```python
from build123d import *

# Parameters (mm, degrees)
F0_R     = 5.375
F0_R_2   = 2.6
F1_DEPTH = 3
F2_DEPTH = 1


with BuildPart() as f1:
    # F0 (on Top) → F1 (new body)
    with BuildSketch(Plane.XY):
        with BuildLine():
            Line((75, 10), (0, 10))
            ThreePointArc((0, 10), (-10, 0), (0, -10))
            Line((0, -10), (75, -10))
            ThreePointArc((75, -10), (85, 0), (75, 10))
        make_face()
        Circle(F0_R, mode=Mode.SUBTRACT)
        with Locations((75, 0)):
            Circle(F0_R, mode=Mode.SUBTRACT)
        with Locations((75, 0)):
            Circle(F0_R)
        with Locations((75, 0)):
            Circle(F0_R_2, mode=Mode.SUBTRACT)
        Circle(F0_R)
        Circle(F0_R_2, mode=Mode.SUBTRACT)
    extrude(amount=-F1_DEPTH)

    # F0 (on Top) → F2 (cut)
    with BuildSketch(Plane.XY):
        with Locations((75, 0)):
            Circle(F0_R)
        with Locations((75, 0)):
            Circle(F0_R_2, mode=Mode.SUBTRACT)
        Circle(F0_R)
        Circle(F0_R_2, mode=Mode.SUBTRACT)
    extrude(amount=-F2_DEPTH, mode=Mode.SUBTRACT)


solid = f1.part
```
Work out the finished part from the listing and answer in its coordinate system (mm). A direction names the side the tool comes from. Coordinates: 2 decimals unless noted, no trailing zeros. Write each loop counter-clockwise with the first axis right and the second up, starting at its lowest first coordinate (ties: lowest second). Pieces come first, ordered by that corner, then holes.
Q1. A cutting plane is placed at C-C, the plane x = 76. Give the vertices of the cut face in (y, z).
Q2. Determine the mould class of faces 1 (the face through (-10, 0, -1)), 2 (the face through (37, -10, -1)), 3 (the face through (-0.7, 5.33, -0.49)), 4 (the face through (80.13, 1.61, -0.49)) for opening direction X: released by +X, released by -X, zero draft, split by the parting line, or undercut.
Q3. Find the intervals of material crossed by line 1 (X direction, y = 1, z = -1.7); line 2 (Y direction, x = 0, z = -2.2); line 3 (Y direction, x = 0, z = -0.3) (3 decimals), in increasing order.
Q4. A cutting plane is placed at B-B, the plane z = -1.9. Give the vertices of the cut face in (x, y).
Q5. Each of these flat-tipped pins is pushed along its axis until it touches: pin 1 Ø6 at (x, y) = (75, 0) entering from +Z; pin 2 Ø1 at (y, z) = (3, -2) entering from -X. Where does it stop, or does it pass through?
Q6. A cutting plane is placed at A-A, the plane y = 0. Give the vertices of the cut face in (x, z) (3 decimals).
Q7. A cutting plane is placed at D-D, the plane y = -8. Give the vertices of the cut face in (x, z).
Q8. Which of the six approach directions +Z, -Z, +X, -X, +Y, -Y give full straight-line access (tool end or side, diameter ignored) to faces 5 (the face through (37, 0, -3)), 6 (the face through (72.5, 1.3, -1))?
Findings below:
1. outline: (-9.95, -3) - (-2.4, -3) - (-2.4, -1) - (-5.28, -1) - (-5.28, 0) - (-9.95, 0) - close; (2.4, -3) - (9.95, -3) - (9.95, 0) - (5.28, 0) - (5.28, -1) - (2.4, -1) - close
2. face 1: released by -X
2. face 2: zero draft
2. face 3: undercut
2. face 4: undercut
3. line 1: x = -9.95 to -2.4, 2.4 to 72.6, 77.4 to 84.95
3. line 2: y = -10 to -2.6, 2.6 to 10
3. line 3: y = -10 to -5.375, 5.375 to 10
4. outline: (0, -10) - (75, -10) arc R10 ccw to (75, 10) - (0, 10) arc R10 ccw to start; hole circle Ø5.2 at (0, 0); hole circle Ø5.2 at (75, 0)
5. pin 1: stops at z = -1
5. pin 2: stops at x = -9.68
6. outline: (-10, -3) - (-2.6, -3) - (-2.6, -1) - (-5.375, -1) - (-5.375, 0) - (-10, 0) - close; (2.6, -3) - (72.4, -3) - (72.4, -1) - (69.625, -1) - (69.625, 0) - (5.375, 0) - (5.375, -1) - (2.6, -1) - close; (77.6, -3) - (85, -3) - (85, 0) - (80.375, 0) - (80.375, -1) - (77.6, -1) - close
7. outline: (-6, -3) - (81, -3) - (81, 0) - (-6, 0) - close
8. face 5: -Z, +X, -X, +Y, -Y
8. face 6: +Z
